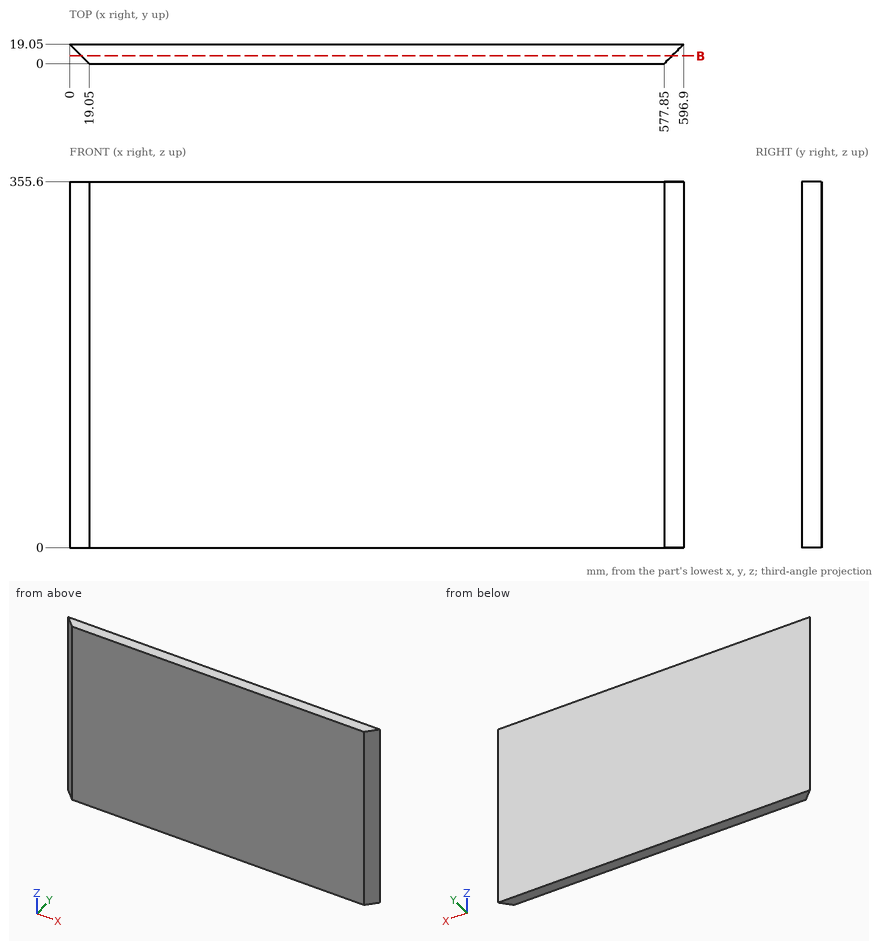
The drawing under review shows one solid part. Ordinate dimensions are in mm from its lowest x, y, z. Coordinates: 2 decimals unless noted, no trailing zeros. Write each loop counter-clockwise with the first axis right and the second up, starting at its lowest first coordinate (ties: lowest second). Pieces come first, ordered by that corner, then holes. Notation, with made-up numbers: (28, 58.5) - (48, 58.5) arc R16 ccw to (48, 70.5) - close; hole circle Ø7 at (53.5, 81.5). An arc over 180 degrees is marked (long way). Use one line per item in the form item = value.
Q1. Consider section B-B (y = 7.5). Write out the cut boundary in (x, z), plus the area to 3 significant figures.
Taken from the geometry:
outline = (11.55, 0) - (585.35, 0) - (585.35, 355.6) - (11.55, 355.6) - close
area = 204,000 mm^2
Q2. Insertion check: pin 1 Ø8 at (x, y) = (460.5, 11.5) entering from -Z; pin 2 Ø5 at (y, z) = (17, 168) entering from -X; pin 3 Ø1 at (y, z) = (10, 151) entering from -X. Each pin has a flat end and moves straight along its axis. Give the tip position at first contact, or say it passes through.
Taken from the geometry:
pin_1 = 0
pin_2 = 0
pin_3 = 8.55
Q3. For probe 1 along X at (y, z) = (3.5, 280.5); probe 2 along X at (y, z) = (9.5, 181), list the stretches that pass through material, from the lowest coordinate up.
Taken from the geometry:
probe_1 = 15.55 to 581.35
probe_2 = 9.55 to 587.35
